Model file for the job. Use its own axes, mm. Give positions to 0.01 mm unless a question says otherwise; leave off trailing zeros. Write each loop counter-clockwise with the first axis right and the second up, starting at its lowest first coordinate (ties: lowest second). Pieces come first, ordered by that corner, then holes.
```python
from build123d import *

# Parameters (mm, degrees)
SKETCH1_W           = 155
SKETCH1_H           = 50
SKETCH1_R           = 9
BOSS_EXTRUDE1_DEPTH = 30


with BuildPart() as part:
    # Sketch1 → Boss-Extrude1 (new body)
    with BuildSketch(Plane(origin=(0, 0, 0), x_dir=(1, 0, 0), z_dir=(0, 1, 0))):
        with Locations((7.5, 5)):
            Rectangle(SKETCH1_W, SKETCH1_H)
        Circle(SKETCH1_R, mode=Mode.SUBTRACT)
    extrude(amount=BOSS_EXTRUDE1_DEPTH)


solid = part.part
```
1. Slice it at A-A, the plane z = 0. Write the cut outline in (x, y).
Calculated:
outline: (-70, 0) - (-9, 0) - (-9, 30) - (-70, 30) - close; (9, 0) - (85, 0) - (85, 30) - (9, 30) - close
2. Probe probe 1 along X at (y, z) = (19.5, 0); probe 2 along Z at (x, y) = (0, 15); probe 3 along X at (y, z) = (25.75, -5.5). List the from-to ranges inside material, lowest first.
Calculated:
probe 1: x = -70 to -9, 9 to 85
probe 2: z = -30 to -9, 9 to 20
probe 3: x = -70 to -7.12, 7.12 to 85
3. Slice it at B-B, the plane y = 26.5. Write the cut outline in (x, z).
Calculated:
outline: (-70, -30) - (85, -30) - (85, 20) - (-70, 20) - close; hole circle Ø18 at (0, 0)
